from build123d import *

# Parameters (mm, degrees)
SKETCH1_R           = 27.5
BOSS_EXTRUDE1_DEPTH = 2
SKETCH2_R           = 29.25
BOSS_EXTRUDE2_DEPTH = 7
SKETCH3_R           = 1.5
CUT_EXTRUDE1_DEPTH  = 65.622944842
CIRPATTERN1_COUNT   = 8
CUT_EXTRUDE2_DEPTH  = 65.622944842
CIRPATTERN2_COUNT   = 8


with BuildPart() as part:
    # Sketch1 → Boss-Extrude1 (new body)
    with BuildSketch(Plane.XY):
        Polygon((-45.25, -18.743163697), (-45.25, 18.743163697), (-18.743163697, 45.25), (18.743163697, 45.25), (45.25, 18.743163697), (45.25, -18.743163697), (18.743163697, -45.25), (-18.743163697, -45.25), align=None)
        Circle(SKETCH1_R, mode=Mode.SUBTRACT)
    extrude(amount=BOSS_EXTRUDE1_DEPTH)

    # Sketch2 → Boss-Extrude2 (add)
    with BuildSketch(Plane.XY.offset(2)):
        Polygon((18.743163697, 45.25), (-18.743163697, 45.25), (-45.25, 18.743163697), (-45.25, -18.743163697), (-18.743163697, -45.25), (18.743163697, -45.25), (45.25, -18.743163697), (45.25, 18.743163697), align=None)
        Circle(SKETCH2_R, mode=Mode.SUBTRACT)
    extrude(amount=BOSS_EXTRUDE2_DEPTH)

    # Sketch3 → Cut-Extrude1 (cut, through all)
    with BuildSketch(Plane(origin=(0, 0, 0), x_dir=(-1, 0, 0), z_dir=(0, 0, -1))):
        with Locations((17.125083598, 41.34360908)):
            Circle(SKETCH3_R)
    cut_extrude1 = extrude(amount=-CUT_EXTRUDE1_DEPTH, mode=Mode.SUBTRACT)

    # CirPattern1: Cut-Extrude1 ×8 about axis
    cirpattern1_axis = Axis((0, 0, 0), (0, 0, 1))
    for i in range(1, CIRPATTERN1_COUNT):
        add(cut_extrude1.rotate(cirpattern1_axis, i * 360 / CIRPATTERN1_COUNT), mode=Mode.SUBTRACT)

    # Sketch6 → Cut-Extrude2 (cut, through all)
    with BuildSketch(Plane.XY.offset(9)):
        Polygon((-10.445300105, 31.75), (10.445300105, 31.75), (12.930581479, 37.75), (-12.930581479, 37.75), align=None)
    cut_extrude2 = extrude(amount=-CUT_EXTRUDE2_DEPTH, mode=Mode.SUBTRACT)

    # CirPattern2: Cut-Extrude2 ×8 about axis
    cirpattern2_axis = Axis((0, 0, 0), (0, 0, 1))
    for i in range(1, CIRPATTERN2_COUNT):
        add(cut_extrude2.rotate(cirpattern2_axis, i * 360 / CIRPATTERN2_COUNT), mode=Mode.SUBTRACT)


solid = part.part
Geometry: final body of the model. Coordinates: model frame, mm. A direction names the side the tool comes from. Coordinates: 2 decimals unless noted, no trailing zeros. Loops run counter-clockwise (first coordinate to the right, second up) from the corner with the lowest first, then second, coordinate; pieces in that order, holes last. Notation, with made-up numbers: (2, -40) - (49, -40) arc R27 ccw to (49, -18) - close; hole circle Ø4 at (6.25, 71.25). An arc over 180 degrees is marked (long way). Put each result on its own line as item: value. Start each with the question number.
Q1. Line query: line 1 (Y direction, x = -0.5, z = 6.5); line 2 (Y direction, x = 10, z = 8); line 3 (X direction, y = -22, z = 0.75). Output: solid intervals per line, ascending.
Q2. Cut plane A-A, the plane y = 0. Return loops of the section in (x, z), and give its area (3 significant figures).
Q3. Cut plane D-D, the plane z = 3.75. Give the number of separate pieces and of enclosed holes in the cut face, and give its area (3 significant figures).
Q4. Set-up query: faces 4 (the flat face through (0, 37.75, 5)), 5 (the flat face through (21, -19, 0)). Return all of +Z, -Z, +X, -X, +Y, -Y with unobstructed straight access to the full face (end or side cutting, diameter ignored); none if empty.
Q5. Pin query (flat end, axial travel): pin 1 Ø3 at (y, z) = (-25, 4.5) entering from +X; pin 2 Ø5 at (x, z) = (-24, 8) entering from -Y. Return the tip coordinate at first contact, or that it passes through.
Q6. Cut plane C-C, the plane y = 34. Return loops of the section in (x, z).
Q7. Pull-direction query (Y, two-part tool) for faces 1 (the flat face through (45.25, 0, 4)), 2 (the flat face through (-31.811, 32.182, 4.437)), 3 (the flat face through (0, -37.75, 5)); classes: released by +Y, released by -Y, zero draft, split by the parting line, or undercut.
Filled sheet:
1. line 1: -45.25 to -37.75, -31.75 to -29.25, 29.25 to 31.75, 37.75 to 45.25
1. line 2: -45.25 to -37.75, -31.75 to -27.49, 27.49 to 31.75, 37.75 to 45.25
1. line 3: -41.99 to -31.39, -22.9 to -16.5, 16.5 to 22.9, 31.39 to 41.99
2. outline: (-45.25, 0) - (-37.75, 0) - (-37.75, 9) - (-45.25, 9) - close; (-31.75, 0) - (-27.5, 0) - (-27.5, 2) - (-29.25, 2) - (-29.25, 9) - (-31.75, 9) - close; (27.5, 0) - (31.75, 0) - (31.75, 9) - (29.25, 9) - (29.25, 2) - (27.5, 2) - close; (37.75, 0) - (45.25, 0) - (45.25, 9) - (37.75, 9) - close
2. area: 187 mm²
3. separate pieces: 1
3. enclosed holes: 17
3. area: 2,920 mm²
4. face 4: +Z, -Z
4. face 5: -Z, +X, -X, +Y, -Y
5. pin 1: x = 40.49
5. pin 2: y = -42.49
6. outline: (-29.99, 0) - (-19.39, 0) - (-19.39, 9) - (-29.99, 9) - close; (-16.79, 0) - (-11.38, 0) - (-11.38, 9) - (-16.79, 9) - close; (11.38, 0) - (16.79, 0) - (16.79, 9) - (11.38, 9) - close; (19.39, 0) - (29.99, 0) - (29.99, 9) - (19.39, 9) - close
7. face 1: zero draft
7. face 2: released by +Y
7. face 3: undercut
